Design review of the part built by this model. Coordinates are the model's own, in mm. A direction names the side the tool comes from. Round coordinates to 2 decimals unless told otherwise and drop trailing zeros. Order: outer loops, then holes, each group sorted by start corner. A loop starts at its lowest first (then second) coordinate and runs counter-clockwise, first axis right, second up. Notation, with made-up numbers: (26.25, 44) - (40.25, 44) arc R33 ccw to (40.25, 79) - close; hole circle Ø6 at (31, 62). An arc over 180 degrees is marked (long way). Use CSV: the item, a comma, the result in double quotes.
from build123d import *

# Parameters (mm, degrees)
F1_DEPTH = 8.2
F2_W     = 7.775
F2_H     = 7.775
F3_DEPTH = 1.8


# Not quite as in the source:
# - a feature names something its author has since deleted; it is built from what else it names


with BuildPart() as f1:
    # F0 (on Top) → F1 (new body)
    with BuildSketch(Plane.XY):
        with BuildLine():
            Line((13.775, 10.775), (13.775, 13.775))
            Line((13.775, 13.775), (10.775, 13.775))
            Line((10.775, 13.775), (11.275, 12.375))
            Line((11.275, 12.375), (8.275, 12.375))
            Line((8.275, 12.375), (8.775, 13.775))
            Line((8.775, 13.775), (0, 13.775))
            Line((0, 13.775), (0, 13.1))
            ThreePointArc((0, 13.1), (9.2630988335, 9.2630988335), (13.1, 0))
            Line((13.1, 0), (13.775, 0))
            Line((13.775, 0), (13.775, 8.775))
            Line((13.775, 8.775), (13.775, 10.775))
        make_face()
        Polygon((15.175, 11.275), (13.775, 10.775), (13.775, 8.775), (15.175, 8.275), align=None)
        Polygon((15.175, -8.275), (13.775, -8.775), (13.775, -10.775), (15.175, -11.275), align=None)
        with BuildLine():
            Line((13.775, -8.775), (13.775, 0))
            Line((13.775, 0), (13.1, 0))
            ThreePointArc((13.1, 0), (12.1028218759, -5.013152964), (9.2630988335, -9.2630988335))
            Line((9.2630988335, -9.2630988335), (13.775, -13.775))
            Line((13.775, -13.775), (13.775, -10.775))
            Line((13.775, -10.775), (13.775, -8.775))
        make_face()
        with BuildLine():
            Line((13.775, -13.775), (9.2630988335, -9.2630988335))
            ThreePointArc((9.2630988335, -9.2630988335), (5.013152964, -12.1028218759), (0, -13.1))
            Line((0, -13.1), (0, -13.775))
            Line((0, -13.775), (8.775, -13.775))
            Line((8.775, -13.775), (10.775, -13.775))
            Line((10.775, -13.775), (13.775, -13.775))
        make_face()
        Polygon((11.275, -15.175), (10.775, -13.775), (8.775, -13.775), (8.275, -15.175), align=None)
        with BuildLine():
            ThreePointArc((0, -13.1), (-9.2630988335, -9.2630988335), (-13.1, 0))
            Line((-13.1, 0), (-13.775, 0))
            Line((-13.775, 0), (-13.775, -8.775))
            Line((-13.775, -8.775), (-12.375, -8.275))
            Line((-12.375, -8.275), (-12.375, -11.275))
            Line((-12.375, -11.275), (-13.775, -10.775))
            Line((-13.775, -10.775), (-13.775, -13.775))
            Line((-13.775, -13.775), (-10.775, -13.775))
            Line((-10.775, -13.775), (-8.775, -13.775))
            Line((-8.775, -13.775), (0, -13.775))
            Line((0, -13.775), (0, -13.1))
        make_face()
        Polygon((-8.275, -15.175), (-8.775, -13.775), (-10.775, -13.775), (-11.275, -15.175), align=None)
        with BuildLine():
            ThreePointArc((-13.1, 0), (-12.1028218759, 5.013152964), (-9.2630988335, 9.2630988335))
            Line((-9.2630988335, 9.2630988335), (-13.775, 13.775))
            Line((-13.775, 13.775), (-13.775, 10.775))
            Line((-13.775, 10.775), (-12.375, 11.275))
            Line((-12.375, 11.275), (-12.375, 8.275))
            Line((-12.375, 8.275), (-13.775, 8.775))
            Line((-13.775, 8.775), (-13.775, 0))
            Line((-13.775, 0), (-13.1, 0))
        make_face()
        with BuildLine():
            Line((0, 13.1), (0, 13.775))
            Line((0, 13.775), (-8.775, 13.775))
            Line((-8.775, 13.775), (-8.275, 12.375))
            Line((-8.275, 12.375), (-9.775, 12.375))
            Line((-9.775, 12.375), (-11.275, 12.375))
            Line((-11.275, 12.375), (-10.775, 13.775))
            Line((-10.775, 13.775), (-13.775, 13.775))
            Line((-13.775, 13.775), (-9.2630988335, 9.2630988335))
            ThreePointArc((-9.2630988335, 9.2630988335), (-5.013152964, 12.1028218759), (0, 13.1))
        make_face()
    extrude(amount=F1_DEPTH)

    # F2 (on face) → F3 (join)
    with BuildSketch(Plane.XY.offset(8.2)):
        Polygon((-6, 13.775), (-13.775, 13.775), (-6, 6), align=None)
        Polygon((-6, -13.775), (-6, -6), (-13.775, -13.775), align=None)
        Polygon((-13.775, -13.775), (-6, -6), (-13.775, -6), align=None)
        Polygon((-6, 6), (-13.775, 13.775), (-13.775, 6), align=None)
        with Locations((9.8875, -9.8875)):
            Rectangle(F2_W, F2_H)
        with Locations((9.8875, 9.8875)):
            Rectangle(F2_W, F2_H)
    extrude(amount=F3_DEPTH)


solid = f1.part
1) The part is to be moulded in two halves that separate along X. For faces 6 (the face through (-0.1, -13.4, 8.2)), 7 (the face through (-11.022, -14.465, 4.043)), 8 (the face through (11.4, -7.1, 0)), say which applies: +X half, -X half, draft (parallel to the pull), parting line (faces both ways), or undercut.
Data:
face 6,"undercut"
face 7,"-X half"
face 8,"draft"
2) We need section D-D (x = -10). Give the boundary of the cut face in (y, z) (3 decimals), then the cut area to 3 significant figures.
Data:
outline,"(-15.175, 0) - (-8.462, 0) - (-8.462, 8.2) - (-6, 8.2) - (-6, 10) - (-13.775, 10) - (-13.775, 8.2) - (-15.175, 8.2) - close; (6, 8.2) - (8.462, 8.2) - (8.462, 0) - (12.375, 0) - (12.375, 8.2) - (13.775, 8.2) - (13.775, 10) - (6, 10) - close"
area,"115 mm2"
3) Insertion check: pin 1 Ø3 at (x, z) = (-3.5, 8) entering from -Y (3 decimals); pin 2 Ø0.9 at (x, z) = (10, 6) entering from +Y (3 decimals); pin 3 Ø0.9 at (y, z) = (10, 2) entering from -X (3 decimals). Each pin has a flat end and moves straight along its axis. Give the tip position at first contact, or say it passes through.
Data:
pin 1,"stops at y = -13.775"
pin 2,"stops at y = 12.375"
pin 3,"stops at x = -12.375"
4) We need section A-A (z = 8.75). Give the boundary of the cut face in (x, y) (3 decimals).
Data:
outline,"(-13.775, -13.775) - (-6, -13.775) - (-6, -6) - (-13.775, -6) - close; (-13.775, 6) - (-6, 6) - (-6, 13.775) - (-13.775, 13.775) - close; (6, -13.775) - (13.775, -13.775) - (13.775, -6) - (6, -6) - close; (6, 6) - (13.775, 6) - (13.775, 13.775) - (6, 13.775) - close"
5) We need section B-B (x = 1.25). Give the boundary of the cut face in (y, z) (3 decimals).
Data:
outline,"(-13.775, 0) - (-13.04, 0) - (-13.04, 8.2) - (-13.775, 8.2) - close; (13.04, 0) - (13.775, 0) - (13.775, 8.2) - (13.04, 8.2) - close"
6) We need section C-C (y = 5). Give the boundary of the cut face in (x, z) (3 decimals).
Data:
outline,"(-13.775, 0) - (-12.108, 0) - (-12.108, 8.2) - (-13.775, 8.2) - close; (12.108, 0) - (13.775, 0) - (13.775, 8.2) - (12.108, 8.2) - close"
7) To check wall thickness, follow L1, parallel to Y at x = -6.25, z = 9.25 (3 decimals); L2, parallel to X at y = 3.25, z = 5.75 (3 decimals); L3, parallel to X at y = 3, z = 7.75 (3 decimals). State the ranges of each line that lie inside material, in increasing order. Write a range as from..to.
Data:
L1,"y = -13.775..-6, 6..13.775"
L2,"x = -13.775..-12.69, 12.69..13.775"
L3,"x = -13.775..-12.752, 12.752..13.775"
8) For faces 1 (the face through (14, -10, 8.2)), 2 (the face through (10, -6, 9)), 3 (the face through (14.465, -11.022, 4.043)), 4 (the face through (14.485, -8.522, 4.043)), 5 (the face through (10, 13, 8.2)), list the 3-axis set-ups (+Z, -Z, +X, -X, +Y, -Y) from which the entire face can be reached by the end or side of a thin tool; tool diameter is ignored.
Data:
face 1,"+Z, +X, +Y, -Y"
face 2,"+Z, +X, -X"
face 3,"+Z, -Z, -Y"
face 4,"+Z, -Z"
face 5,"-Z"
